Geometry: see drawing. Coordinates: mm, zero at the bounding-box minimum. A direction names the side the tool comes from. Give positions to 0.01 mm unless a question says otherwise; leave off trailing zeros. Loops run counter-clockwise (first coordinate to the right, second up) from the corner with the lowest first, then second, coordinate; pieces in that order, holes last. Notation, with made-up numbers: (65, 35.25) -> (109, 35.25) arc R27 ccw to (109, 71.25) -> close; hole circle Ø7 at (-17, 72.25). An arc over 180 degrees is marked (long way). Return JSON: item names as keys, results as strings. Group by question number.
(1) Cut plane B-B on z = 21. Return loops of the section in (x, y), then the cut area to 3 significant figures.
(2) Draft query along X for the marked faces 3, 4 and 5. Return one class per face: released by +X, released by -X, zero draft, split by the parting line, or undercut.
(3) Cut plane D-D on x = 32. Return loops of the section in (y, z), then the cut area to 3 significant figures.
(4) Access query for the marked faces 1 and 2. Directions: +Z, -Z, +X, -X, +Y, -Y. A direction counts if a zero-diameter tool reaches every point of the face in a straight line with its end or side. Return the directions, or none.
(5) Ray query, line 1 (Y direction, x = 45, z = 30); line 2 (Z direction, x = 22.5, y = 26.75); line 3 (Y direction, x = 45, z = 48). Return the intervals inside material, ascending. Write a range as from..to.
(6) Pin query (flat end, axial travel): pin 1 (4 mm diameter, centred on y = 21, z = 53, fed in from -X); pin 2 (2 mm diameter, centred on x = 31.5, z = 36, fed in from -Y); pin 3 (10 mm diameter, centred on y = 20.5, z = 52, fed in from -X). Return the tip coordinate at first contact, or that it passes through.
(7) Cut plane C-C on y = 15. Return loops of the section in (x, z), then the cut area to 3 significant figures.
(8) Cut plane A-A on x = 45. Return loops of the section in (y, z), then the cut area to 3 significant figures.
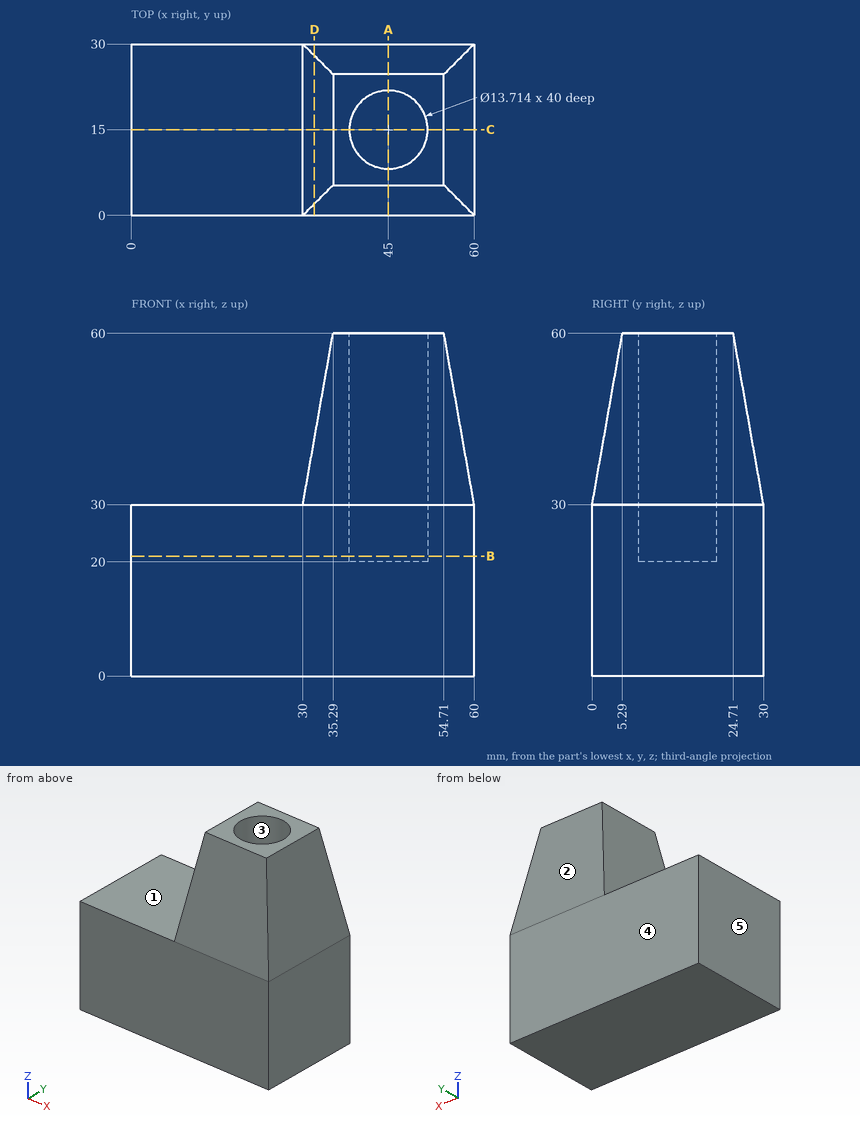
Answers:
{
 "1": {"outline": "(0, 0) -> (60, 0) -> (60, 30) -> (0, 30) -> close; hole circle Ø13.71 at (45, 15)", "area": "1,650 mm²"},
 "2": {"face 3": "undercut", "face 4": "zero draft", "face 5": "released by -X"},
 "3": {"outline": "(0, 0) -> (30, 0) -> (30, 30) -> (28, 41.34) -> (2, 41.34) -> (0, 30) -> close", "area": "1,220 mm²"},
 "4": {"face 1": "+Z, -X, +Y, -Y", "face 2": "+Z, +X, -X, +Y"},
 "5": {"line 1": "0..8.14, 21.86..30", "line 2": "0..30", "line 3": "3.17..8.14, 21.86..26.83"},
 "6": {"pin 1": "x = 33.7", "pin 2": "y = 0.88", "pin 3": "x = 33"},
 "7": {"outline": "(0, 0) -> (60, 0) -> (60, 30) -> (54.71, 60) -> (51.86, 60) -> (51.86, 20) -> (38.14, 20) -> (38.14, 60) -> (35.29, 60) -> (30, 30) -> (0, 30) -> close", "area": "1,990 mm²"},
 "8": {"outline": "(0, 0) -> (30, 0) -> (30, 30) -> (24.71, 60) -> (21.86, 60) -> (21.86, 20) -> (8.14, 20) -> (8.14, 60) -> (5.29, 60) -> (0, 30) -> close", "area": "1,090 mm²"}
}
